Read the model definition and answer for the solid it produces. Units are mm, in the model's axes. Face numbers are marked on the shaded views. A direction names the side the tool comes from. Round coordinates to 2 decimals unless told otherwise and drop trailing zeros. Write each loop counter-clockwise with the first axis right and the second up, starting at its lowest first coordinate (ties: lowest second). Pieces come first, ordered by that corner, then holes. Notation, with made-up numbers: (25.25, 81.25) -> (43.25, 81.25) arc R8 ccw to (43.25, 92.25) -> close; hole circle Ø1 at (33, 65.5). An arc over 180 degrees is marked (long way). Return JSON: item names as keys, results as strings.
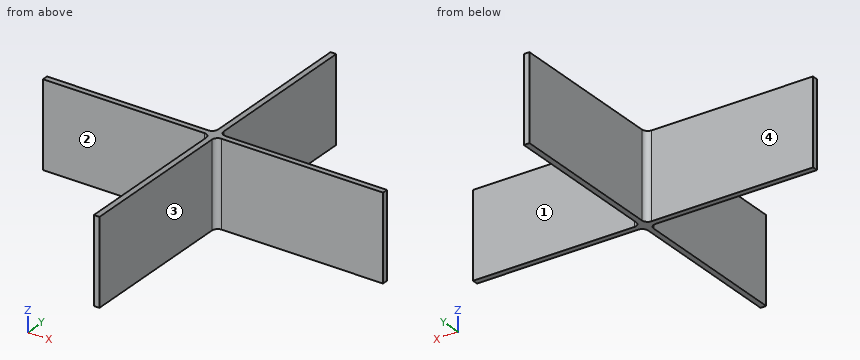
from build123d import *

# Parameters (mm, degrees)
F0_W     = 149.86
F0_H     = 5.08
F0_W_2   = 2.54
F1_DEPTH = 76.2
F2_R     = 5.08


with BuildPart() as f1:
    # F0 (on Top) → F1 (new body)
    with BuildSketch(Plane.XY):
        with Locations((74.93, -2.54)):
            Rectangle(F0_W, F0_H)
        Polygon((149.86, 149.86), (149.86, 0), (152.4, 0), (154.94, 0), (154.94, 149.86), align=None)
        with Locations((229.87, -2.54)):
            Rectangle(F0_W, F0_H)
        with Locations((151.13, -2.54)):
            Rectangle(F0_W_2, F0_H)
        with Locations((153.67, -2.54)):
            Rectangle(F0_W_2, F0_H)
        Polygon((152.4, -5.08), (149.86, -5.08), (149.86, -154.94), (154.94, -154.94), (154.94, -5.08), align=None)
    extrude(amount=F1_DEPTH)

    # F2
    f2_edges = [f1.edges().sort_by_distance(p)[0] for p in [
        (149.86, -5.08, 38.1),
        (154.94, -5.08, 38.1),
        (154.94, 0, 38.1),
        (149.86, 0, 38.1),
    ]]
    fillet(f2_edges, radius=F2_R)


solid = f1.part
Item 1: Section B-B (x = 233.5) is taken. Give the vertices of the cut face in (y, z).
Worked answers:
{"outline": "(-5.08, 0) -> (0, 0) -> (0, 76.2) -> (-5.08, 76.2) -> close"}
Item 2: Flat-ended cylindrical pins translate along their axes: pin 1 (3 mm diameter, centred on y = 50.5, z = 39, fed in from -X); pin 2 (8 mm diameter, centred on x = 99, z = 52.5, fed in from -Y); pin 3 (23 mm diameter, centred on y = -115.5, z = 26, fed in from +X); pin 4 (12 mm diameter, centred on x = 145, y = -109, fed in from +Z). Find the tip coordinate at first contact, or state that the pin passes through.
Worked answers:
{"pin 1": "stops at x = 149.86", "pin 2": "stops at y = -5.08", "pin 3": "stops at x = 154.94", "pin 4": "stops at z = 76.2"}
Item 3: A tool of negligible diameter and unlimited length cuts with its end or side. For the marked faces 1, 2, 3 and 4, from which of +Z, -Z, +X, -X, +Y, -Y can it reach the whole face along a straight path? Write none if from no direction.
Worked answers:
{"face 1": "+Z, -Z, +X, +Y", "face 2": "+Z, -Z, -X, -Y", "face 3": "+Z, -Z, +X, -Y", "face 4": "+Z, -Z, -X, +Y"}
Item 4: Section A-A (z = 19) is taken. Give the vertices of the cut face in (x, y).
Worked answers:
{"outline": "(0, -5.08) -> (144.78, -5.08) arc R5.08 cw to (149.86, -10.16) -> (149.86, -154.94) -> (154.94, -154.94) -> (154.94, -10.16) arc R5.08 cw to (160.02, -5.08) -> (304.8, -5.08) -> (304.8, 0) -> (160.02, 0) arc R5.08 cw to (154.94, 5.08) -> (154.94, 149.86) -> (149.86, 149.86) -> (149.86, 5.08) arc R5.08 cw to (144.78, 0) -> (0, 0) -> close"}
Item 5: Straight lines are drawn through the part: L1, parallel to X at y = 99, z = 4; L2, parallel to Y at x = 54.5, z = 73; L3, parallel to Y at x = 146, z = 64. For each, find the intervals that lie inside material, in ascending order. Write a range as [from, to].
Worked answers:
{"L1": "x = [149.86, 154.94]", "L2": "y = [-5.08, 0]", "L3": "y = [-5.23, 0.15]"}
Item 6: Section C-C (y = -77) is taken. Give the vertices of the cut face in (x, z), then the cut area to 3 significant figures.
Worked answers:
{"outline": "(149.86, 0) -> (154.94, 0) -> (154.94, 76.2) -> (149.86, 76.2) -> close", "area": "387 mm2"}
